CAD build for the part. Positions are in the model's coordinates, mm. Round coordinates to 2 decimals unless told otherwise and drop trailing zeros. Loops run counter-clockwise (first coordinate to the right, second up) from the corner with the lowest first, then second, coordinate; pieces in that order, holes last. Notation, with made-up numbers: M 42,23.5 L 61,23.5 A11 cw 61,37.5 Z; hole C 5.25,-35 d5. An arc over 180 degrees is marked long. Use a Markdown table: item, result. Add a question column.
(1) Flat gauge pins, fed straight in: P1, Ø4, axis at y = -11, z = -9.5, coming from the -X side; P2, Ø3, axis at x = -2, z = 10.5, coming from the +Y side; P3, Ø8, axis at x = 4.5, y = 4, coming from the -Z side; P4, Ø1.5, axis at x = 7.5, z = 10, coming from the -Y side. Where does each tip first touch, or does it go through?
(2) Band-saw the part on B-B, the plane y = 10.5. Write the cut outline in (x, z), and give its area (3 significant figures).
(3) Band-saw the part on A-A, the plane y = 5. Write the cut outline in (x, z).
(4) Wall check: L1, parallel to X at y = 1.5, z = -2; L2, parallel to Z at x = 3.75, y = -13.5; L3, parallel to Y at x = 10, z = -9.25. Give the ranges that are in metal, low to high.
from build123d import *


with BuildPart() as part:
    # Esboço1 → Revolução1 (revolve)
    with BuildSketch(Plane.XY):
        with BuildLine():
            Line((1.016555702, -17.534294806), (1.016555702, 16.265705194))
            ThreePointArc((1.016555702, 16.265705194), (2.06121806, 15.973437857), (2.553565234, 15.006828371))
            ThreePointArc((2.553565234, 15.006828371), (2.92828475, 9.651459509), (3.433565234, 4.306828371))
            ThreePointArc((3.433565234, 4.306828371), (5.268808127, -0.263802551), (9.433565234, -2.893171629))
            ThreePointArc((9.433565234, -2.893171629), (12.192236118, -3.637403975), (14.933565234, -4.443171629))
            ThreePointArc((14.933565234, -4.443171629), (15.258578175, -5.111100137), (14.721555702, -5.624294806))
            ThreePointArc((14.721555702, -5.624294806), (12.658414234, -6.31213617), (10.621555702, -7.074294806))
            ThreePointArc((10.621555702, -7.074294806), (8.276967202, -8.358909194), (6.486555702, -10.344294806))
            ThreePointArc((6.486555702, -10.344294806), (4.488079996, -13.598838615), (2.336555702, -16.754294806))
            ThreePointArc((2.336555702, -16.754294806), (1.76887547, -17.300528258), (1.016555702, -17.534294806))
        make_face()
    revolve(axis=Axis((1.016555702, -17.534294806, 0), (0, 1, 0)))


solid = part.part
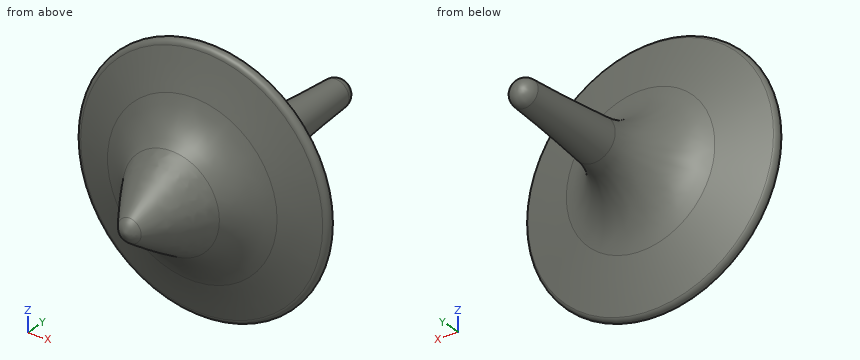
Return value:
| question | item | result |
|---|---|---|
| 1 | P1 | through |
| 1 | P2 | y = -3.16 |
| 1 | P3 | z = -3.35 |
| 1 | P4 | y = -6.48 |
| 2 | outline | C 1.02,0 d3.69 |
| 2 | area | 10.7 mm^2 |
| 3 | outline | C 1.02,0 d4.69 |
| 4 | L1 | -1.4 to 3.43 |
| 4 | L2 | -2.24 to 2.24 |
| 4 | L3 | -5.88 to -4.13 |
